Autodesk Inventor part; units mm, degrees
ref_plane "YZ Plane" through (0, 0, 0) normal (1, 0, 0) x (0, 1, 0)
ref_plane "XZ Plane" through (0, 0, 0) normal (0, 1, 0) x (-1, 0, 0)
ref_plane "XY Plane" through (0, 0, 0) normal (0, 0, 1) x (1, 0, 0)
sketch "Sketch1" plane through (0, 0, 0) normal (1, 0, 0) x (0, 1, 0)
  line L0 (19.05, 0) -> (-19.05, 0) construction
  circle A0 centre (19.05, 0) radius 2.54
  circle A1 centre (-19.05, 0) radius 2.54
  circle A2 centre (0, -34.925) radius 4.064
  line L1 (0, 0) -> (0, -34.925) construction
  arc A3 (27.412, -4.5611) -> (19.05, 9.525) centre (19.05, 0) ccw
  arc A4 (-19.05, 9.525) -> (-27.412, -4.5611) centre (-19.05, 0) ccw
  arc A5 (-8.362, -39.4861) -> (8.362, -39.4861) centre (0, -34.925) ccw
  line L2 (-8.362, -39.4861) -> (-27.412, -4.5611)
  line L3 (-19.05, 9.525) -> (19.05, 9.525)
  line L4 (27.412, -4.5611) -> (8.362, -39.4861)
  dimension "d0" = 5.08
  dimension "d2" = 38.1
  dimension "d3" = 8.128
  dimension "d4" = 34.925
  dimension "d5" = 9.525
extrude "Extrusion1" add sketch "Sketch1" along normal blind 3.175
properties part number "roller plate" material "Aluminum 6061"
Check sheet for the modelled part. Datum: model origin and axes. Units: mm. Give positions to 0.01 mm unless a question says otherwise; leave off trailing zeros. Loops run counter-clockwise (first coordinate to the right, second up) from the corner with the lowest first, then second, coordinate; pieces in that order, holes last. Notation, with made-up numbers: M -8.75,-28.5 L 48.25,-28.5 A29 cw 48.25,-0.5 Z; hole C 2,23 d9. An arc over 180 degrees is marked long. Answer in a Markdown table with one row per item.
1) Depth check by flat-ended pin: pin 1 (1.5 mm diameter, centred on x = 2, z = -34.5, fed in from +Y); pin 2 (1 mm diameter, centred on x = 1.5, y = 11, fed in from -Z). Enter the tip coordinate at first touch or a pass-through.
Solutions:
| item | result |
|---|---|
| pin 1 | stops at y = 11.49 |
| pin 2 | stops at z = -35.57 |
2) Thickness scan on line 1 (Z direction, x = 3, y = 2) (3 decimals); line 2 (Y direction, x = 2.85, z = 1); line 3 (Z direction, x = 1.9, y = -19.05) (3 decimals). Record the ranges inside material, lowest first.
Solutions:
| item | result |
|---|---|
| line 1 | z = -44.238 to -38.463, -31.387 to 9.525 |
| line 2 | y = -28.52 to -21.38, -16.72 to 16.72, 21.38 to 28.52 |
| line 3 | z = -19.891 to -2.54, 2.54 to 9.525 |
3) Cross-section at B-B (y = 0). Enter the section's corners in (x, z) (3 decimals).
Solutions:
| item | result |
|---|---|
| outline | M 0,-44.45 L 3.175,-44.45 L 3.175,-38.989 L 0,-38.989 Z; M 0,-30.861 L 3.175,-30.861 L 3.175,9.525 L 0,9.525 Z |
4) Mould release check, pull along Y, two halves, no side actions. Record for faces 1 (the face through (1.57, 27.17, 4.98)), 2 (the face through (1.57, -19.38, -2.52)), 3 (the face through (1.6, 17, 1.5)), 4 (the face through (0, 0, -11)): released by +Y, released by -Y, zero draft, split by the parting line, or undercut.
Solutions:
| item | result |
|---|---|
| face 1 | released by +Y |
| face 2 | undercut |
| face 3 | undercut |
| face 4 | zero draft |
5) Cross-section at D-D (y = 13.5). Enter the section's corners in (x, z) (3 decimals).
Solutions:
| item | result |
|---|---|
| outline | M 0,-30.066 L 3.175,-30.066 L 3.175,9.525 L 0,9.525 Z |
6) Cross-section at A-A (z = 0). Enter the section's corners in (x, y) (3 decimals).
Solutions:
| item | result |
|---|---|
| outline | M 0,-28.575 L 3.175,-28.575 L 3.175,-21.59 L 0,-21.59 Z; M 0,-16.51 L 3.175,-16.51 L 3.175,16.51 L 0,16.51 Z; M 0,21.59 L 3.175,21.59 L 3.175,28.575 L 0,28.575 Z |
7) Cross-section at C-C (x = 2.55). Enter the section's corners in (y, z) (3 decimals), plus the area to 3 significant figures.
Solutions:
| item | result |
|---|---|
| outline | M -27.412,-4.561 L -8.362,-39.486 A9.525 ccw 8.362,-39.486 L 27.412,-4.561 A9.525 ccw 19.05,9.525 L -19.05,9.525 A9.525 ccw Z; hole C -19.05,0 d5.08; hole C 0,-34.925 d8.128; hole C 19.05,0 d5.08 |
| area | 1,980 mm^2 |
